Study the drawing (mm; zero at the part's minimum x, y, z) and answer. A direction names the side the tool comes from. Coordinates: 2 decimals unless noted, no trailing zeros. Order: outer loops, then holes, each group sorted by start corner. A loop starts at its lowest first (then second) coordinate and runs counter-clockwise, first axis right, second up. Notation, with made-up numbers: (36.25, -8.75) -> (94.25, -8.75) arc R15 ccw to (94.25, -1.75) -> close; hole circle Ø1 at (58.5, -23.5). An arc over 180 degrees is marked (long way). Write each question's results on one line, items separated by ' | '. Start each with the question number.
(1) The part is cut by section A-A, the plane x = 825. Give the vertices of the cut face in (y, z).
(2) A tool of negligible diameter and unlimited length cuts with its end or side. For the marked faces 1 and 2, from which of +Z, -Z, +X, -X, +Y, -Y can it reach the whole face along a straight path? Write none if from no direction.
(3) Straight lines are drawn through the part: L1, parallel to Y at x = 75, z = 361; L2, parallel to Z at x = 690.5, y = 162; L3, parallel to X at y = 40.5, z = 295. For each, find the intervals that lie inside material, in ascending order.
(4) Determine the mould class of the marked faces 3, 4 and 5 for opening direction Z: +Z half, -Z half, draft (parallel to the pull), parting line (faces both ways), or undercut.
(5) The part is cut by section B-B, the plane z = 360. Give the vertices of the cut face in (x, y), then the cut area to 3 significant figures.
(6) The part is cut by section D-D, the plane y = 235. Give the vertices of the cut face in (x, z), then the cut area to 3 significant figures.
(7) Given pin 1 (15 mm diameter, centred on y = 37.5, z = 143.5, fed in from -X); pin 2 (15 mm diameter, centred on y = 32.5, z = 186, fed in from +X), each flat-ended and moving along its own axis, determine where each tip first touches the part or whether it passes through.
(8) The part is cut by section C-C, the plane y = 150. Give the vertices of the cut face in (x, z).
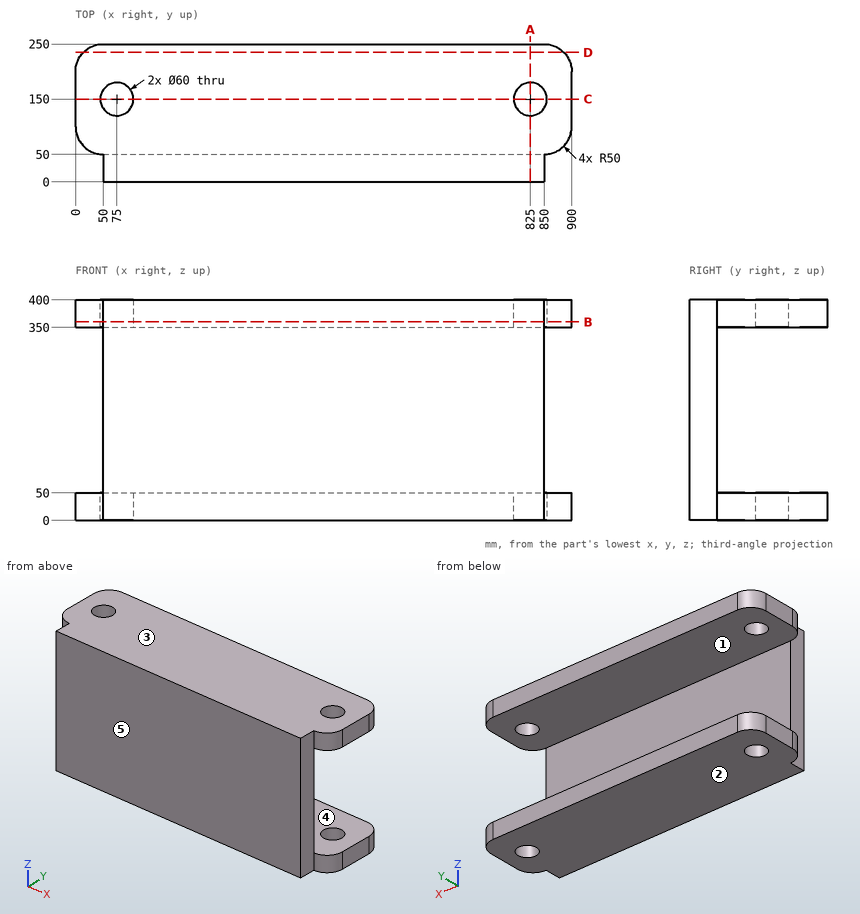
Established:
1) outline: (0, 0) -> (120, 0) -> (120, 50) -> (50, 50) -> (50, 350) -> (120, 350) -> (120, 400) -> (0, 400) -> close; (180, 0) -> (250, 0) -> (250, 50) -> (180, 50) -> close; (180, 350) -> (250, 350) -> (250, 400) -> (180, 400) -> close
2) face 1: +X, -X, +Y | face 2: -Z, +X, -X, +Y, -Y
3) L1: y = 0 to 120, 180 to 250 | L2: z = 0 to 50, 350 to 400 | L3: x = 50 to 850
4) face 3: +Z half | face 4: undercut | face 5: draft
5) outline: (0, 100) arc R50 ccw to (50, 50) -> (50, 0) -> (850, 0) -> (850, 50) arc R50 ccw to (900, 100) -> (900, 200) arc R50 ccw to (850, 250) -> (50, 250) arc R50 ccw to (0, 200) -> close; hole circle Ø60 at (75, 150); hole circle Ø60 at (825, 150) | area: 212,000 mm^2
6) outline: (14.29, 0) -> (885.71, 0) -> (885.71, 50) -> (14.29, 50) -> close; (14.29, 350) -> (885.71, 350) -> (885.71, 400) -> (14.29, 400) -> close | area: 87,100 mm^2
7) pin 1: stops at x = 50 | pin 2: stops at x = 850
8) outline: (0, 0) -> (45, 0) -> (45, 50) -> (0, 50) -> close; (0, 350) -> (45, 350) -> (45, 400) -> (0, 400) -> close; (105, 0) -> (795, 0) -> (795, 50) -> (105, 50) -> close; (105, 350) -> (795, 350) -> (795, 400) -> (105, 400) -> close; (855, 0) -> (900, 0) -> (900, 50) -> (855, 50) -> close; (855, 350) -> (900, 350) -> (900, 400) -> (855, 400) -> close
